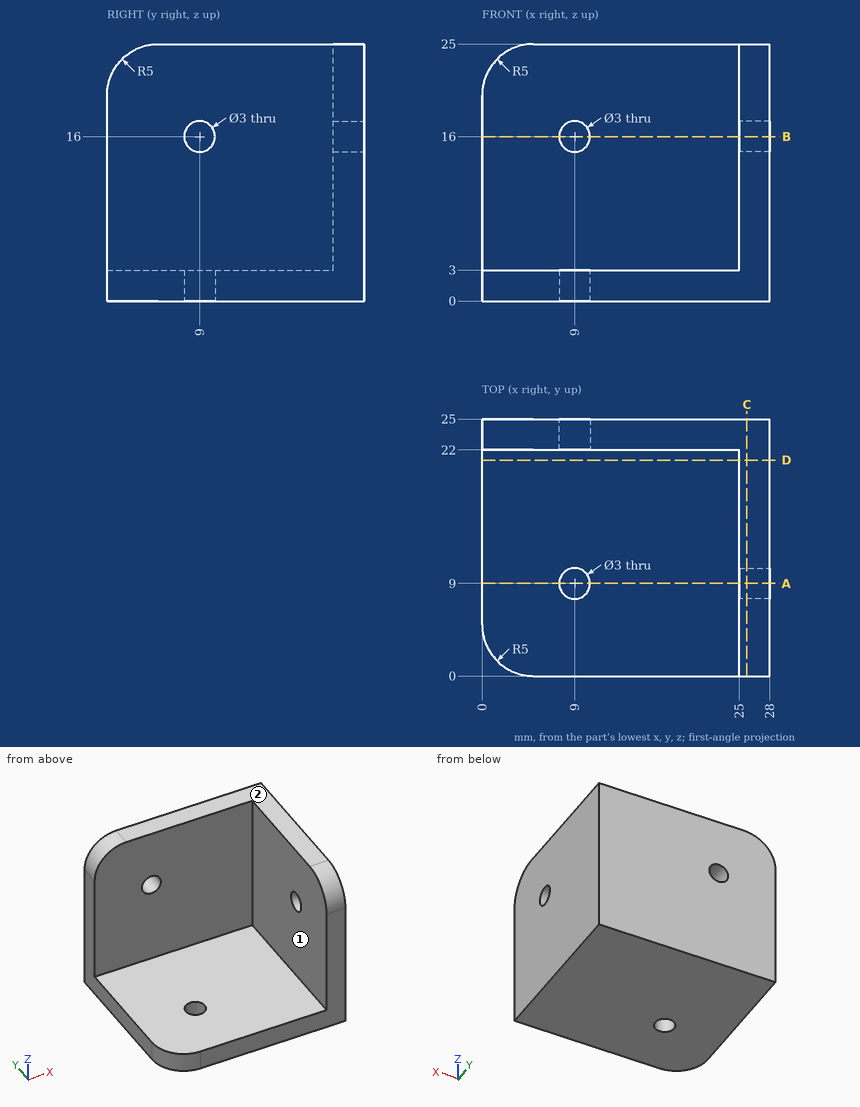
Design review of the part shown in the three views and the two pictorial views. Dimensions are in mm from the part's minimum x, y and z. A direction names the side the tool comes from. Coordinates: 2 decimals unless noted, no trailing zeros. Write each loop counter-clockwise with the first axis right and the second up, starting at its lowest first coordinate (ties: lowest second). Pieces come first, ordered by that corner, then holes.
1) We need section A-A on y = 9. State the section outline as (x, z) points, then the cut area to 3 significant figures.
2) We need section D-D on y = 21. State the section outline as (x, z) points, then the cut area to 3 significant figures.
3) We need section C-C on x = 25.75. State the section outline as (y, z) points, then the cut area to 3 significant figures.
4) We need section B-B on z = 16. State the section outline as (x, y) points.
5) To check wall thickness, follow probe 1 along Y at (x, z) = (9, 1); probe 2 along X at (y, z) = (20.25, 22.25); probe 3 along Z at (x, y) = (17.5, 19). State the ranges of each line that lie inside material, in increasing order.
6) Machinability: for the marked faces 1 and 2, which of the approach directions +Z, -Z, +X, -X, +Y, -Y give a long, thin tool a straight path to every point of the face, cutting with its end or side? Answer none if there is none.
7) Clearance check with flat-ended pins moving along their axes: pin 1 Ø3.5 at (x, z) = (9, 16) entering from -Y; pin 2 Ø1.5 at (y, z) = (4, 11.5) entering from -X; pin 3 Ø11 at (x, y) = (13, 11) entering from +Z; pin 4 Ø2.5 at (y, z) = (9, 16) entering from +X. State where each tip first meets the part, or that it passes through.
Answer list:
1. outline: (0, 0) - (7.5, 0) - (7.5, 3) - (0, 3) - close; (10.5, 0) - (28, 0) - (28, 14.5) - (25, 14.5) - (25, 3) - (10.5, 3) - close; (25, 17.5) - (28, 17.5) - (28, 25) - (25, 25) - close
1. area: 132 mm2
2. outline: (0, 0) - (28, 0) - (28, 25) - (25, 25) - (25, 3) - (0, 3) - close
2. area: 150 mm2
3. outline: (0, 0) - (25, 0) - (25, 25) - (5, 25) arc R5 ccw to (0, 20) - close; hole circle Ø3 at (9, 16)
3. area: 613 mm2
4. outline: (0, 22) - (7.5, 22) - (7.5, 25) - (0, 25) - close; (10.5, 22) - (25, 22) - (25, 10.5) - (28, 10.5) - (28, 25) - (10.5, 25) - close; (25, 0) - (28, 0) - (28, 7.5) - (25, 7.5) - close
5. probe 1: y = 0 to 7.5, 10.5 to 25
5. probe 2: x = 25 to 28
5. probe 3: z = 0 to 3
6. face 1: +Z, -X, -Y
6. face 2: +Z, +X, -X, +Y, -Y
7. pin 1: stops at y = 22
7. pin 2: stops at x = 25
7. pin 3: stops at z = 3
7. pin 4: passes through
